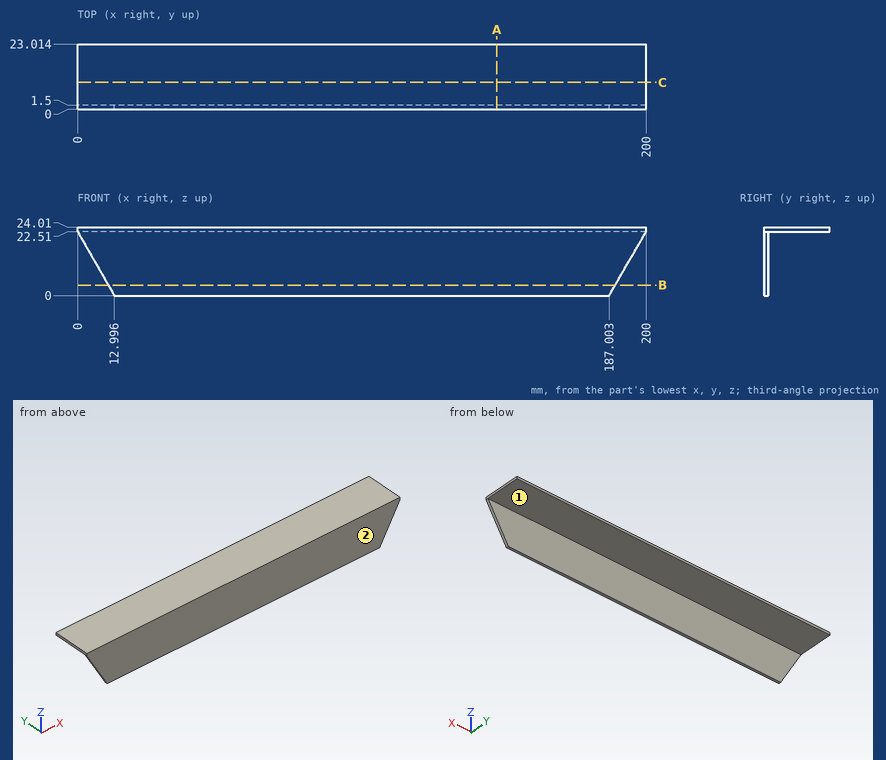
Source: three-view drawing plus pictorial views. Frame: mm from the lowest corner of the part. A direction names the side the tool comes from. Give positions to 0.01 mm unless a question says otherwise; leave off trailing zeros. Order: outer loops, then holes, each group sorted by start corner. A loop starts at its lowest first (then second) coordinate and runs counter-clockwise, first axis right, second up. Notation, with made-up numbers: (40.25, 30.5) -> (76.25, 30.5) arc R20 cw to (76.25, 51.5) -> close; hole circle Ø3 at (10, 46). An arc over 180 degrees is marked (long way). Write each question's results on one line, items separated by ' | '. Start each with the question number.
Item 1: Cut plane B-B on z = 3.75. Return the cut outline in (x, y).
Item 2: Set-up query: the marked faces 1 and 2. Return all of +Z, -Z, +X, -X, +Y, -Y with unobstructed straight access to the full face (end or side cutting, diameter ignored); none if empty.
Item 3: Line query: line 1 (Y direction, x = 140.5, z = 6.25); line 2 (Z direction, x = 25, y = 3.25). Output: solid intervals per line, ascending.
Item 4: Cut plane C-C on y = 9.5. Return the cut outline in (x, z), then the cut area to 3 significant figures.
Item 5: Contact query for flat-ended pins moving along their axis: P1, Ø6, axis at x = 60, z = 11.5, coming from the +Y side; P2, Ø6, axis at y = 2.5, z = 20.5, coming from the +X side. Output: stop coordinate, or through.
Item 6: Cut plane A-A on x = 147.5. Return the cut outline in (y, z) (1 decimal).
Established:
1) outline: (10.83, 0) -> (189.17, 0) -> (189.17, 1.5) -> (10.83, 1.5) -> close
2) face 1: -Z, +X, -X, +Y | face 2: +Z, -Z, +X, -X, -Y
3) line 1: 0 to 1.5 | line 2: 22.51 to 24.01
4) outline: (0, 22.51) -> (200, 22.51) -> (200, 24.01) -> (0, 24.01) -> close | area: 300 mm^2
5) P1: y = 1.5 | P2: x = 200
6) outline: (0, 0) -> (1.5, 0) -> (1.5, 22.5) -> (23, 22.5) -> (23, 24) -> (0, 24) -> close
